Build history of the part. All positions in model axes, mm. A direction names the side the tool comes from. Round coordinates to 2 decimals unless told otherwise and drop trailing zeros. Loops run counter-clockwise (first coordinate to the right, second up) from the corner with the lowest first, then second, coordinate; pieces in that order, holes last. Notation, with made-up numbers: (39, 38.25) -> (82, 38.25) arc R34 ccw to (82, 72.25) -> close; hole circle Ø1 at (-33.75, 24.25). An arc over 180 degrees is marked (long way). Put each result on its own line as item: value. Start each with the question number.
Item 1: Tool access for faces 1 (the flat face through (-3.75, -16, -6)), 2 (the flat face through (-12.25, -2, -7)), 3 (the flat face through (8, -13, -6.5)): list every direction of +Z, -Z, +X, -X, +Y, -Y with a clear straight run to the whole face (end or side of a thin tool).
Item 2: Cut at B-B, the plane y = 5. List the corners of the cut face in (x, z), plus the area to 3 significant figures.
Item 3: Flat gauge pins, fed straight in: pin 1 Ø5 at (x, y) = (0, -7) entering from -Z; pin 2 Ø1.5 at (x, z) = (4.5, -6) entering from -Y; pin 3 Ø1.2 at (x, y) = (8, -12.5) entering from -Z; pin 4 Ø1.5 at (x, y) = (3, 4.5) entering from -Z. Where does each tip first touch, or does it go through?
Item 4: Cut at A-A, the plane x = 0. List the corners of the cut face in (y, z).
Item 5: Drill centre lines: probe 1 along X at (y, z) = (5, 1.25); probe 2 along X at (y, z) = (8.5, -5.25); probe 3 along Y at (x, z) = (0, 1.75). Where is each one in solid material? Low to high. Write a range as [from, to].
Item 6: Pull direction Y, two halves, no side cores. Call faces 4 (the cylindrical face through (0, -4, 2)), 5 (the flat face through (0, 13, 1)), 6 (the cylindrical face through (-0.08, -17.743, 0.246)): +Y half, -Y half, draft (parallel to the pull), parting line (faces both ways), or undercut.
Item 7: Cut at D-D, the plane y = -7. List the corners of the cut face in (x, z), plus the area to 3 significant figures.
Item 8: Cut at C-C, the plane z = -6. List the corners of the cut face in (x, y).
```python
from build123d import *

# Parameters (mm, degrees)
SKETCH1_W           = 20.5
SKETCH1_H           = 30.25
SKETCH1_R           = 1.3
SKETCH1_R_2         = 3
BOSS_EXTRUDE1_DEPTH = 3.5
SKETCH2_W           = 2
SKETCH2_H           = 18.5
BOSS_EXTRUDE2_DEPTH = 30.25
SKETCH3_W           = 6.5
SKETCH3_H           = 10.5
BOSS_EXTRUDE3_DEPTH = 2
FILLET1_R           = 3.5
FILLET2_R           = 2
SKETCH4_R           = 2.25
CUT_EXTRUDE1_DEPTH  = 1.5
FILLET4_R           = 3
SKETCH9_W           = 4
SKETCH9_H           = 4
BOSS_EXTRUDE4_DEPTH = 6.5
FILLET6_R           = 1.5
BOSS_EXTRUDE5_DEPTH = 2
BOSS_EXTRUDE6_DEPTH = 1


with BuildPart() as part:
    # Sketch1 → Boss-Extrude1 (new body)
    with BuildSketch(Plane.XY):
        with Locations((0, -2.125)):
            Rectangle(SKETCH1_W, SKETCH1_H)
        with Locations((-4.8, 5)):
            Circle(SKETCH1_R, mode=Mode.SUBTRACT)
        with Locations((4.8, 5)):
            Circle(SKETCH1_R, mode=Mode.SUBTRACT)
        with Locations((0, -7)):
            Circle(SKETCH1_R_2, mode=Mode.SUBTRACT)
    extrude(amount=BOSS_EXTRUDE1_DEPTH)

    # Sketch2 → Boss-Extrude2 (add)
    with BuildSketch(Plane(origin=(0, -17.25, 0), x_dir=(-1, 0, 0), z_dir=(0, -1, 0))):
        with Locations((11.25, 5.75)):
            Rectangle(SKETCH2_W, SKETCH2_H)
        with Locations((-11.25, 5.75)):
            Rectangle(SKETCH2_W, SKETCH2_H)
    extrude(amount=-BOSS_EXTRUDE2_DEPTH)

    # Sketch3 → Boss-Extrude3 (add)
    with BuildSketch(Plane.XZ.offset(17.25)):
        with Locations((-7, -5.25)):
            Rectangle(SKETCH3_W, SKETCH3_H)
        with Locations((7, -5.25)):
            Rectangle(SKETCH3_W, SKETCH3_H)
    extrude(amount=-BOSS_EXTRUDE3_DEPTH)

    # Fillet1
    fillet1_edges = [part.edges().sort_by_distance(p)[0] for p in [
        (-3.75, -16.25, 0),
        (3.75, -16.25, 0),
    ]]
    fillet(fillet1_edges, radius=FILLET1_R)

    # Fillet2
    fillet2_edges = [part.edges().sort_by_distance(p)[0] for p in [
        (-12.25, -2.125, 3.5),
        (12.25, -2.125, 3.5),
    ]]
    fillet(fillet2_edges, radius=FILLET2_R)

    # Sketch4 → Cut-Extrude1 (cut)
    with BuildSketch(Plane.XY.offset(3.5)):
        with Locations((-4.8, 5)):
            Circle(SKETCH4_R)
        with Locations((4.8, 5)):
            Circle(SKETCH4_R)
    extrude(amount=-CUT_EXTRUDE1_DEPTH, mode=Mode.SUBTRACT)

    # Fillet4
    fillet4_edges = [part.edges().sort_by_distance(p)[0] for p in [
        (-11.25, 13, -15),
        (-11.25, -17.25, -15),
        (11.25, 13, -15),
        (11.25, -17.25, -15),
    ]]
    fillet(fillet4_edges, radius=FILLET4_R)

    # Sketch9 → Boss-Extrude4 (add)
    with BuildSketch(Plane(origin=(0, 0, 0), x_dir=(-1, 0, 0), z_dir=(0, 0, -1))):
        with Locations((-8.25, -13.25)):
            Rectangle(SKETCH9_W, SKETCH9_H)
        with Locations((8.25, -13.25)):
            Rectangle(SKETCH9_W, SKETCH9_H)
    extrude(amount=BOSS_EXTRUDE4_DEPTH)

    # Fillet6
    fillet6_edges = [part.edges().sort_by_distance(p)[0] for p in [
        (-6.25, -11.25, -3.25),
        (6.25, -11.25, -3.25),
        (-10.25, -16.25, -10.5),
        (10.25, -16.25, -10.5),
        (-3.75, -16.25, -10.5),
        (3.75, -16.25, -10.5),
    ]]
    fillet(fillet6_edges, radius=FILLET6_R)

    # Sketch10 → Boss-Extrude5 (add)
    with BuildSketch(Plane.XZ.offset(17.25)):
        with BuildLine():
            Line((-0.25, 0), (0.25, 0))
            ThreePointArc((0.25, 0), (2.668052064, -0.969580229), (3.746392428, -3.341129019))
            Line((3.746392428, -3.341129019), (1.948302942, -3.341129019))
            ThreePointArc((1.948302942, -3.341129019), (0, -1.545230361), (-1.948302942, -3.341129019))
            Line((-1.948302942, -3.341129019), (-3.746392428, -3.341129019))
            ThreePointArc((-3.746392428, -3.341129019), (-2.668052064, -0.969580229), (-0.25, 0))
        make_face()
    extrude(amount=-BOSS_EXTRUDE5_DEPTH)

    # Sketch11 → Boss-Extrude6 (add)
    with BuildSketch(Plane.XZ.offset(17.25)):
        with BuildLine():
            Line((-1.948302942, -3.341129019), (-3.746392428, -3.341129019))
            ThreePointArc((-3.746392428, -3.341129019), (0, 0.246607561), (3.746392428, -3.341129019))
            Line((3.746392428, -3.341129019), (1.948302942, -3.341129019))
            ThreePointArc((1.948302942, -3.341129019), (0, -1.545230361), (-1.948302942, -3.341129019))
        make_face()
    extrude(amount=BOSS_EXTRUDE6_DEPTH)


solid = part.part
```
Reply:
1. face 1: -Z, +Y, -Y
1. face 2: +Z, -Z, -X, +Y, -Y
1. face 3: -Z, +Y
2. outline: (-12.25, -15) -> (-10.25, -15) -> (-10.25, 0) -> (-6.1, 0) -> (-6.1, 2) -> (-7.05, 2) -> (-7.05, 3.5) -> (-10.25, 3.5) arc R2 ccw to (-12.25, 1.5) -> close; (-3.5, 0) -> (3.5, 0) -> (3.5, 2) -> (2.55, 2) -> (2.55, 3.5) -> (-2.55, 3.5) -> (-2.55, 2) -> (-3.5, 2) -> close; (6.1, 0) -> (10.25, 0) -> (10.25, -15) -> (12.25, -15) -> (12.25, 1.5) arc R2 ccw to (10.25, 3.5) -> (7.05, 3.5) -> (7.05, 2) -> (6.1, 2) -> close
2. area: 120 mm^2
3. pin 1: passes through
3. pin 2: stops at y = -17.25
3. pin 3: stops at z = -6.5
3. pin 4: stops at z = 0
4. outline: (-18.25, -1.55) -> (-15.25, -1.55) -> (-15.25, 0) -> (-10, 0) -> (-10, 3.5) -> (-17.25, 3.5) -> (-17.25, 0.25) -> (-18.25, 0.25) -> close; (-4, 0) -> (13, 0) -> (13, 3.5) -> (-4, 3.5) -> close
5. probe 1: x = [-12.25, -6.1], [-3.5, 3.5], [6.1, 12.25]
5. probe 2: x = [-12.25, -10.25], [10.25, 12.25]
5. probe 3: y = [-17.25, -10], [-4, 13]
6. face 4: undercut
6. face 5: +Y half
6. face 6: draft
7. outline: (-12.25, -15) -> (-10.25, -15) -> (-10.25, 0) -> (-3, 0) -> (-3, 3.5) -> (-10.25, 3.5) arc R2 ccw to (-12.25, 1.5) -> close; (3, 0) -> (10.25, 0) -> (10.25, -15) -> (12.25, -15) -> (12.25, 1.5) arc R2 ccw to (10.25, 3.5) -> (3, 3.5) -> close
7. area: 123 mm^2
8. outline: (-12.25, -17.25) -> (-3.75, -17.25) -> (-3.75, -15.25) -> (-6.25, -15.25) -> (-6.25, -12.75) arc R1.5 ccw to (-7.75, -11.25) -> (-10.25, -11.25) -> (-10.25, 13) -> (-12.25, 13) -> close; (3.75, -17.25) -> (12.25, -17.25) -> (12.25, 13) -> (10.25, 13) -> (10.25, -11.25) -> (7.75, -11.25) arc R1.5 ccw to (6.25, -12.75) -> (6.25, -15.25) -> (3.75, -15.25) -> close
